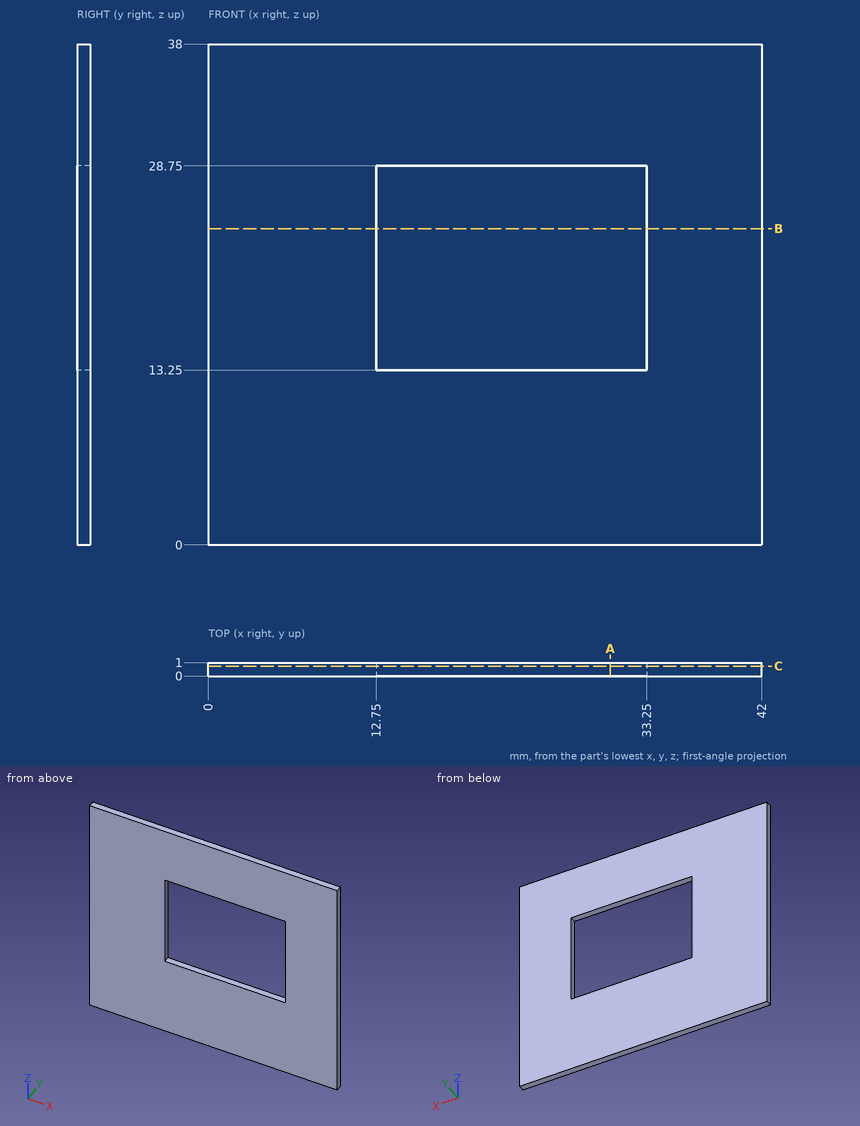
Here's the drawing with two shaded views (mm, measured from the low corner). I have some questions. Round coordinates to 2 decimals unless told otherwise and drop trailing zeros. Loops run counter-clockwise (first coordinate to the right, second up) from the corner with the lowest first, then second, coordinate; pieces in that order, holes last. Notation, with made-up numbers: (8.25, 56.5) - (43.25, 56.5) arc R13 cw to (43.25, 66.5) - close; hole circle Ø7 at (-30.5, -1.5). An arc over 180 degrees is marked (long way). Use CSV: the item, a comma, the result in double quotes. Start each with the question number.
1) If we section it at A-A on x = 30.5: Write out the boundary of the cut face in (y, z).
2) If we section it at C-C on y = 0.75: Write out the boundary of the cut face in (x, z).
3) If we section it at B-B on z = 24: Write out the boundary of the cut face in (x, y), plus the area to 3 significant figures.
4) For pin 1 Ø4 at (x, z) = (23.5, 17) entering from -Y, with a flat end and sliding along its axis, tell me the tip position at first contact or that it passes through.
5) Please list where these lines run through material, in increasing order: probe 1 along Z at (x, y) = (26, 0.85); probe 2 along X at (y, z) = (0.4, 18). Write a range as [from, to].
Geometry results:
1,outline,"(0, 0) - (1, 0) - (1, 13.25) - (0, 13.25) - close; (0, 28.75) - (1, 28.75) - (1, 38) - (0, 38) - close"
2,outline,"(0, 0) - (42, 0) - (42, 38) - (0, 38) - close; hole (12.75, 13.25) - (33.25, 13.25) - (33.25, 28.75) - (12.75, 28.75) - close"
3,outline,"(0, 0) - (12.75, 0) - (12.75, 1) - (0, 1) - close; (33.25, 0) - (42, 0) - (42, 1) - (33.25, 1) - close"
3,area,"21.5 mm2"
4,pin 1,"passes through"
5,probe 1,"z = [0, 13.25], [28.75, 38]"
5,probe 2,"x = [0, 12.75], [33.25, 42]"
